```python
from build123d import *

# Parameters (mm, degrees)
SKETCH1_W                = 15
SKETCH1_H                = 60
BOSS_EXTRUDE2_DEPTH      = 39.11
BOSS_EXTRUDE3_DEPTH      = 12
BOSS_EXTRUDE3_DEPTH_BACK = 27
SKETCH3_W                = 60
SKETCH3_H                = 5
RIB1_REACH               = 55.008
SKETCH5_WALL_W           = 127.334599132
SKETCH5_WALL_H           = 10
SKETCH6_R                = 1.5
CUT_EXTRUDE2_DEPTH       = 50.434219929
SKETCH7_W                = 16
SKETCH7_H                = 16
CUT_EXTRUDE3_DEPTH       = 57.201353187
SKETCH8_R                = 1.75
CUT_EXTRUDE4_DEPTH       = 75.228310637
FILLET1_R                = 3


with BuildPart() as part:
    # Sketch1 → Boss-Extrude2 (new body)
    with BuildSketch(Plane(origin=(0, 0, 0), x_dir=(1, 0, 0), z_dir=(0, 1, 0))):
        Rectangle(SKETCH1_W, SKETCH1_H)
    extrude(amount=BOSS_EXTRUDE2_DEPTH)

    # Sketch3 → Boss-Extrude3 (add, two sides: drawn at the far end of the back side and taken through both)
    with BuildSketch(Plane.ZY.offset(7.5).offset(-BOSS_EXTRUDE3_DEPTH_BACK)):
        with Locations((0, 2.5)):
            Rectangle(SKETCH3_W, SKETCH3_H)
    extrude(amount=BOSS_EXTRUDE3_DEPTH + BOSS_EXTRUDE3_DEPTH_BACK)

    # Sketch5 wall → Rib1 (add, up to next)
    with BuildSketch(Plane(origin=(-12.037058369, 13.5275, 0), x_dir=(-0.46970610176, -0.882822846311, 0), z_dir=(0.882822846311, -0.46970610176, 0)), mode=Mode.PRIVATE) as rib1_sk1:
        Rectangle(SKETCH5_WALL_W, SKETCH5_WALL_H)
    rib1_tool1 = extrude(rib1_sk1.sketch, amount=RIB1_REACH, mode=Mode.PRIVATE) - part.part
    rib1 = rib1_tool1.solids().sort_by_distance((-12.037058369, 13.5275, 0))[0]
    add(rib1)

    # Sketch6 → Cut-Extrude2 (cut, through all)
    with BuildSketch(Plane(origin=(0, 5, 0), x_dir=(1, 0, 0), z_dir=(0, 1, 0))):
        with Locations(Location((-14.5, -25, 0), (0, 0, 270))):
            Circle(SKETCH6_R)
        with Locations(Location((-14.5, 25, 0), (0, 0, 90))):
            Circle(SKETCH6_R)
    cut_extrude2 = extrude(amount=-CUT_EXTRUDE2_DEPTH, mode=Mode.SUBTRACT)

    # Mirror1: Rib1, Cut-Extrude2 across plane
    add(rib1.mirror(Plane(origin=(0, 0, 0), x_dir=(0, 0, 1), z_dir=(1, 0, 0))))
    add(cut_extrude2.mirror(Plane(origin=(0, 0, 0), x_dir=(0, 0, 1), z_dir=(1, 0, 0))), mode=Mode.SUBTRACT)

    # Sketch7 → Cut-Extrude3 (cut, through all)
    with BuildSketch(Plane.ZY.offset(7.5)):
        with Locations((15, 31.11)):
            Rectangle(SKETCH7_W, SKETCH7_H)
    cut_extrude3 = extrude(amount=-CUT_EXTRUDE3_DEPTH, mode=Mode.SUBTRACT)

    # Mirror2: Cut-Extrude3 across plane
    add(cut_extrude3.mirror(Plane.XY), mode=Mode.SUBTRACT)

    # Sketch8 → Cut-Extrude4 (cut, through all)
    with BuildSketch(Plane(origin=(0, 0, -30), x_dir=(-1, 0, 0), z_dir=(0, 0, -1))):
        with Locations(Location((0, 31.61, 0), (0, 0, 90))):
            Circle(SKETCH8_R)
    extrude(amount=-CUT_EXTRUDE4_DEPTH, mode=Mode.SUBTRACT)

    # Fillet1
    fillet1_edges = [part.edges().sort_by_distance(p)[0] for p in [
        (7.5, 5, 17.5),
        (-7.5, 5, -17.5),
        (-7.5, 5, 17.5),
        (-16.574116738, 5, 0),
        (7.5, 5, -17.5),
        (16.574116738, 5, 0),
    ]]
    fillet(fillet1_edges, radius=FILLET1_R)
    fillet1_2_edges = [part.edges().sort_by_distance(p)[0] for p in [
        (19.5, 2.5, -30),
        (19.5, 2.5, 30),
        (-19.5, 2.5, -30),
        (-19.5, 2.5, 30),
    ]]
    fillet(fillet1_2_edges, radius=FILLET1_R)


solid = part.part
```
The model under review builds one solid part; all positions refer to its coordinate system, in mm. A direction names the side the tool comes from. Round coordinates to 2 decimals unless told otherwise and drop trailing zeros. Order: outer loops, then holes, each group sorted by start corner. A loop starts at its lowest first (then second) coordinate and runs counter-clockwise, first axis right, second up. Notation, with made-up numbers: M -20.75,20 L 13.25,20 A27 ccw 13.25,39 Z; hole C 55.25,35.5 d6. An arc over 180 degrees is marked long. Use a Markdown table: item, result.
1) Consider section B-B (z = -25). Write out the cut boundary in (x, y), then the cut area to 3 significant figures.
Report:
| item | result |
|---|---|
| outline | M -19.5,0 L -16,0 L -16,5 L -19.5,5 Z; M -13,0 L 13,0 L 13,5 L 10.5,5 A3 cw 7.5,8 L 7.5,39.11 L -7.5,39.11 L -7.5,8 A3 cw -10.5,5 L -13,5 Z; M 16,0 L 19.5,0 L 19.5,5 L 16,5 Z; hole C 0,31.61 d3.5 |
| area | 671 mm^2 |
2) Draft analysis for pull direction Z (two halves, no side actions). For faces 1 (the face through (11, 10, 5)), 2 (the face through (18.6, 2.54, -29.14)), 3 (the face through (0, 23.11, -15)), 4 (the face through (-19.5, 3, 0)), state which applies: released by +Z, released by -Z, zero draft, split by the parting line, or undercut.
Report:
| item | result |
|---|---|
| face 1 | released by +Z |
| face 2 | released by -Z |
| face 3 | undercut |
| face 4 | zero draft |
3) Consider section A-A (y = 31.61). Write out the cut boundary in (x, z).
Report:
| item | result |
|---|---|
| outline | M -7.5,-30 L -1.75,-30 L -1.75,-23 L -7.5,-23 Z; M -7.5,-7 L -1.75,-7 L -1.75,7 L -7.5,7 Z; M -7.5,23 L -1.75,23 L -1.75,30 L -7.5,30 Z; M 1.75,-30 L 7.5,-30 L 7.5,-23 L 1.75,-23 Z; M 1.75,-7 L 7.5,-7 L 7.5,7 L 1.75,7 Z; M 1.75,23 L 7.5,23 L 7.5,30 L 1.75,30 Z |
4) Tool access review of faces 5 (the face through (-11, 10, -5)), 6 (the face through (-8.4, 5.86, 17.32)), 7 (the face through (8.4, 5.86, -17.68)), 8 (the face through (0, 23.11, 15)): name each direction out of +Z, -Z, +X, -X, +Y, -Y from which nothing blocks a thin tool from reaching the whole face with its end or side.
Report:
| item | result |
|---|---|
| face 5 | -Z, -X, +Y |
| face 6 | +Z, -X, +Y |
| face 7 | -Z, +X, +Y |
| face 8 | +X, -X, +Y |
5) Insertion check: pin 1 (4.5 mm diameter, centred on x = -13.5, z = -6, fed in from +Y); pin 2 (1 mm diameter, centred on x = 9.5, z = 3.5, fed in from +Y); pin 3 (10 mm diameter, centred on x = 13, z = 1.5, fed in from +Y). Each pin has a flat end and moves straight along its axis. Give the tip position at first contact, or say it passes through.
Report:
| item | result |
|---|---|
| pin 1 | y = 14.57 |
| pin 2 | y = 19.24 |
| pin 3 | y = 21.12 |
6) Wall thickness on line 1 along Z through (x, y) = (14.5, 1.4); line 2 along Z through (x, y) = (-4.5, 35.5); line 3 along X through (y, z) = (2, 25): over which ranges is each line inside the solid? List them lowest first. Write a range as [from, to].
Report:
| item | result |
|---|---|
| line 1 | [-30, -26.5], [-23.5, 23.5], [26.5, 30] |
| line 2 | [-30, -23], [-7, 7], [23, 30] |
| line 3 | [-19.5, -16], [-13, 13], [16, 19.5] |
7) Consider section D-D (z = 1.5). Write out the cut boundary in (x, y) (3 decimals).
Report:
| item | result |
|---|---|
| outline | M -19.5,0 L 19.5,0 L 19.5,5 L 18.376,5 A3 cw 15.728,6.591 L 7.5,22.055 L 7.5,39.11 L -7.5,39.11 L -7.5,22.055 L -15.728,6.591 A3 cw -18.376,5 L -19.5,5 Z; hole C 0,31.61 d3.5 |
8) Consider section C-C (x = 0). Write out the cut boundary in (y, z).
Report:
| item | result |
|---|---|
| outline | M 0,-30 L 29.86,-30 L 29.86,-23 L 23.11,-23 L 23.11,-7 L 29.86,-7 L 29.86,7 L 23.11,7 L 23.11,23 L 29.86,23 L 29.86,30 L 0,30 Z; M 33.36,-30 L 39.11,-30 L 39.11,-23 L 33.36,-23 Z; M 33.36,-7 L 39.11,-7 L 39.11,7 L 33.36,7 Z; M 33.36,23 L 39.11,23 L 39.11,30 L 33.36,30 Z |
